Answer from the drawing. Dimensions are ordinates in mm from the lowest x, y and z of the part. Give positions to 0.01 mm unless a question says otherwise; leave off trailing zeros. Order: outer loops, then holes, each group sorted by start corner. A loop starts at its lowest first (then second) coordinate and runs counter-clockwise, first axis right, second up. Notation, with made-up numbers: (73, 88.25) - (110, 88.25) arc R36 ccw to (110, 125.25) - close; hole circle Ø4 at (7.25, -25). An arc over 180 degrees is marked (long way). Answer in a Markdown table with one row per item.
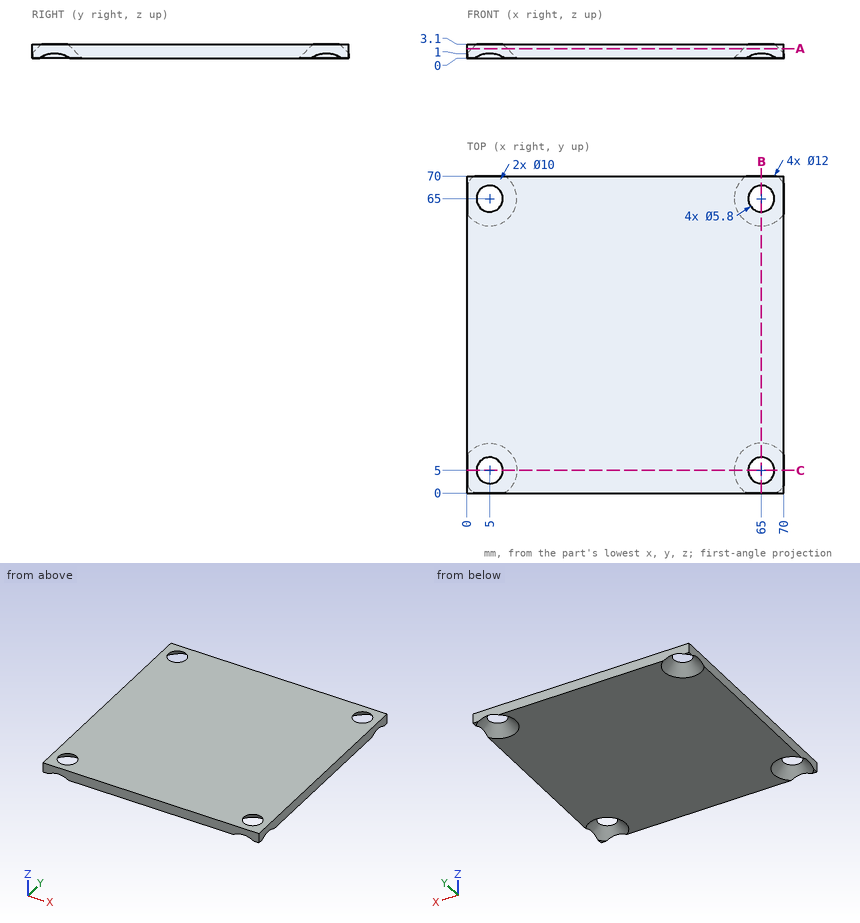
Item 1: Consider line 1 (X direction, y = 8, z = 1.1); line 2 (Z direction, x = 67.5, y = 8); line 3 (X direction, y = 7, z = 0.3). Determine where each line is inside the solid, lowest interval first.
Answer block:
| item | result |
|---|---|
| line 1 | 0 to 1.13, 8.87 to 61.13, 68.87 to 70 |
| line 2 | 2.09 to 3.1 |
| line 3 | 10.34 to 59.66 |
Item 2: Find section B-B on x = 65. Write down the section's boundary in (y, z), then the cut area to 3 significant figures.
Answer block:
| item | result |
|---|---|
| outline | (0, 1) - (2.1, 3.1) - (0, 3.1) - close; (7.9, 3.1) - (11, 0) - (59, 0) - (62.1, 3.1) - close; (67.9, 3.1) - (70, 1) - (70, 3.1) - close |
| area | 163 mm² |
Item 3: Find section A-A on z = 2.1. Write down the section's boundary in (x, y), then the cut area to 3 significant figures.
Answer block:
| item | result |
|---|---|
| outline | (0, 0) - (70, 0) - (70, 70) - (0, 70) - close; hole circle Ø7.8 at (5, 5); hole circle Ø7.8 at (5, 65); hole circle Ø7.8 at (65, 5); hole circle Ø7.8 at (65, 65) |
| area | 4,710 mm² |
